from build123d import *

# Parameters (mm, degrees)
CROQUIS1_R              = 23.6
SALIENTE_EXTRUIR1_DEPTH = 80
VACIADO1_T              = 5
CORTAR_EXTRUIR1_START   = -214
CROQUIS2_R              = 23.6
CORTAR_EXTRUIR1_DEPTH   = 214


with BuildPart() as part:
    # Croquis1 → Saliente-Extruir1 (new body)
    with BuildSketch(Plane(origin=(0, 0, 0), x_dir=(0, 0, -1), z_dir=(1, 0, 0))):
        with BuildLine():
            Line((165, -35), (165, 35))
            ThreePointArc((165, 35), (150.355339059, 70.355339059), (115, 85))
            add(Edge.make_bspline(
                [(-115, 85), (0, 45), (115, 85)],
                knots=[0, 0, 0, 1, 1, 1], degree=2))
            ThreePointArc((-115, 85), (-150.355339059, 70.355339059), (-165, 35))
            Line((-165, 35), (-165, -35))
            ThreePointArc((-165, -35), (-150.355339059, -70.355339059), (-115, -85))
            add(Edge.make_bspline(
                [(-115, -85), (0, -45), (115, -85)],
                knots=[0, 0, 0, 1, 1, 1], degree=2))
            ThreePointArc((115, -85), (150.355339059, -70.355339059), (165, -35))
        make_face()
        with Locations((-100, 0)):
            Circle(CROQUIS1_R, mode=Mode.SUBTRACT)
        with Locations((103.1, 0)):
            Circle(CROQUIS1_R, mode=Mode.SUBTRACT)
    extrude(amount=SALIENTE_EXTRUIR1_DEPTH)

    # Vaciado1
    vaciado1_openings = [part.faces().sort_by_distance(p)[0] for p in [
        (80, 0, 0.122383932),
    ]]
    offset(amount=VACIADO1_T, openings=vaciado1_openings, kind=Kind.INTERSECTION)

    # Croquis2 → Cortar-Extruir1 (cut)
    with BuildSketch(Plane(origin=(80, 0, 0), x_dir=(0, 0, -1), z_dir=(1, 0, 0)).offset(CORTAR_EXTRUIR1_START)):
        with Locations((-100, 0)):
            Circle(CROQUIS2_R)
        with Locations((103.1, 0)):
            Circle(CROQUIS2_R)
    extrude(amount=CORTAR_EXTRUIR1_DEPTH, mode=Mode.SUBTRACT)


solid = part.part
Can you work these out from the model? Positions are in its coordinate system, mm. A direction names the side the tool comes from. Give positions to 0.01 mm unless a question says otherwise; leave off trailing zeros. Loops run counter-clockwise (first coordinate to the right, second up) from the corner with the lowest first, then second, coordinate; pieces in that order, holes last. Notation, with made-up numbers: (83, 13.25) - (134, 13.25) arc R19 cw to (134, 26.25) - close; hole circle Ø8 at (59.5, 69.5). An arc over 180 degrees is marked (long way). Answer as a JSON object with one key per item and string values.
Q1. If I drill on L1, parallel to Z at x = -2, y = 0; L2, parallel to Z at x = 34, y = 10; L3, parallel to X at y = -29, z = -56, over which ranges is the centre line in solid material (lowest first)?
Geometry says:
{"L1": "-170 to -126.7, -79.5 to 76.4, 123.6 to 170", "L2": "-170 to -165, 165 to 170", "L3": "-5 to 0"}
Q2. Imagine slicing it at B-B on y = 60. Write out the boundary of the cut face in (x, z), plus the area to 3 significant figures.
Geometry says:
{"outline": "(-5, -163.99) - (80, -163.99) - (80, -158.3) - (0, -158.3) - (0, 158.3) - (80, 158.3) - (80, 163.99) - (-5, 163.99) - close", "area": "2,550 mm²"}
Q3. Imagine slicing it at A-A on y = 0. Write out the boundary of the cut face in (x, z).
Geometry says:
{"outline": "(-5, -170) - (80, -170) - (80, -165) - (0, -165) - (0, -126.7) - (-5, -126.7) - close; (-5, -79.5) - (0, -79.5) - (0, 76.4) - (-5, 76.4) - close; (-5, 123.6) - (0, 123.6) - (0, 165) - (80, 165) - (80, 170) - (-5, 170) - close"}
Q4. If we mould it in two halves opening along Y, with no side actions, what happens to faces 1 (the flat face through (-5, 1, 2)), 2 (the cylindrical face through (36.9, 73.76, -154.02)), 3 (the cylindrical face through (39.44, -69.964, 150.742)), 4 (the flat face through (0, 1, 2))? For each: pulls with the +Y half, pulls with the -Y half, needs draft (parallel to the pull), parting line crosses it, or undercut.
Geometry says:
{"face 1": "needs draft", "face 2": "pulls with the +Y half", "face 3": "undercut", "face 4": "undercut"}
Q5. Which directions (+Z, -Z, +X, -X, +Y, -Y) give clear straight access to the entire face, cutting with the end or side of a thin tool? Please do faces 5 (the flat face through (37, 0, -170)), 6 (the flat face through (39, 0, -165)).
Geometry says:
{"face 5": "-Z, +X, -X, +Y, -Y", "face 6": "+X"}
Q6. Will these pins go through, and if not, where does the flat tip stop? P1, Ø1, axis at x = 58.5, z = -49.5, coming from the +Y side; P2, Ø5, axis at y = -48, z = 111.5, coming from the +X side; P3, Ø3, axis at x = 28.5, y = 66, coming from the +Z side.
Geometry says:
{"P1": "y = 73.84", "P2": "x = 0", "P3": "z = 161.42"}
